Check sheet for the modelled part. Datum: model origin and axes. Units: mm. Give positions to 0.01 mm unless a question says otherwise; leave off trailing zeros. Write each loop counter-clockwise with the first axis right and the second up, starting at its lowest first coordinate (ties: lowest second). Pieces come first, ordered by that corner, then holes. Notation, with made-up numbers: M -29,74 L -5,74 A27 ccw -5,103 Z; hole C 41,81.5 d9. An arc over 180 degrees is marked long. Write item = value, one per line. Start each with the question number.
1) Scan lines: L1, parallel to X at y = 32, z = 0.1; L2, parallel to Y at x = 0, z = 0.8; L3, parallel to Y at x = -15, z = 0.35. Record each from-to range of solid material in increasing order.
2) Sectioned sample at A-A, the plane y = 14.5. Record the cut outline in (x, z), then the cut area to 3 significant figures.
3) Gauge pin test, flat ends, axial feed: pin 1 (1 mm diameter, centred on y = 5, z = 2, fed in from -X); pin 2 (1 mm diameter, centred on y = 59.5, z = 0.5, fed in from +X); pin 3 (0.9 mm diameter, centred on y = -57, z = 1.5, fed in from -X). Record the tip position at first contact, or that the pin passes through.
4) Sectioned sample at B-B, the plane x = -6. Record the cut outline in (y, z).
from build123d import *

# Parameters (mm, degrees)
F0_R     = 50
F1_DEPTH = 3


with BuildPart() as f1:
    # F0 (on Top) → F1 (new body)
    with BuildSketch(Plane.XY):
        Polygon((16.18034, 63.244295), (0, 75), (-16.18034, 63.244295), (-13.241414, 59.19921), (-15.506661, 57.553411), (-18.445587, 61.598496), (-52.883651, 36.577778), (-49.944725, 32.532693), (-52.209973, 30.886895), (-55.148899, 34.93198), (-71.329239, 23.176275), (-65.148899, 4.155144), (-60.393616, 5.700229), (-59.528369, 3.037271), (-64.283651, 1.492186), (-51.129481, -38.992186), (-46.374199, -37.447101), (-45.508951, -40.110059), (-50.264234, -41.655144), (-44.083894, -60.676275), (-24.083894, -60.676275), (-24.083894, -55.676275), (-21.283894, -55.676275), (-21.283894, -60.676275), (21.283894, -60.676275), (21.283894, -55.676275), (24.083894, -55.676275), (24.083894, -60.676275), (44.083894, -60.676275), (50.264234, -41.655144), (45.508951, -40.110059), (46.374199, -37.447101), (51.129481, -38.992186), (64.283651, 1.492186), (59.528369, 3.037271), (60.393616, 5.700229), (65.148899, 4.155144), (71.329239, 23.176275), (55.148899, 34.93198), (52.209973, 30.886895), (49.944725, 32.532693), (52.883651, 36.577778), (18.445587, 61.598496), (15.506661, 57.553411), (13.241414, 59.19921), align=None)
        Circle(F0_R, mode=Mode.SUBTRACT)
    extrude(amount=F1_DEPTH)


solid = f1.part
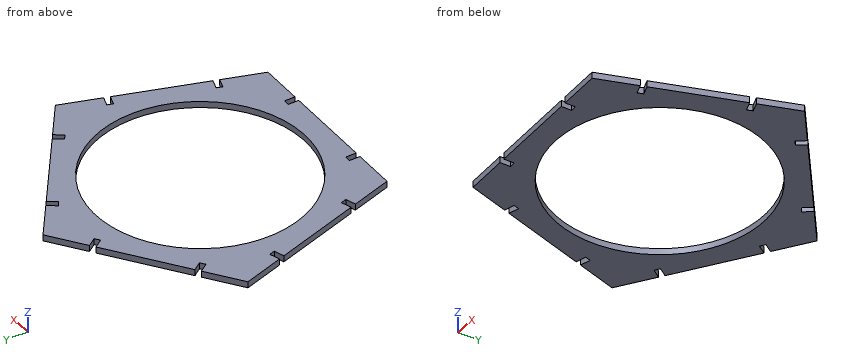
Data:
q1.L1 = -59.18 to -53.02, -50.68 to -38.42, 38.42 to 50.68, 53.02 to 59.18
q1.L2 = -60.68 to -50, 50 to 75
q1.L3 = -60.68 to -47.7, 47.7 to 57.92, 61.62 to 64.1
q2.outline = M -68.51,0 L -47.85,0 L -47.85,3 L -68.51,3 Z; M 47.85,0 L 68.51,0 L 68.51,3 L 47.85,3 Z
q2.area = 124 mm2
q3.pin_1 = -65.59
q3.pin_2 = 22.02
q3.pin_3 = -45.42
q4.outline = M -60.68,0 L -49.64,0 L -49.64,3 L -60.68,3 Z; M 49.64,0 L 70.64,0 L 70.64,3 L 49.64,3 Z
